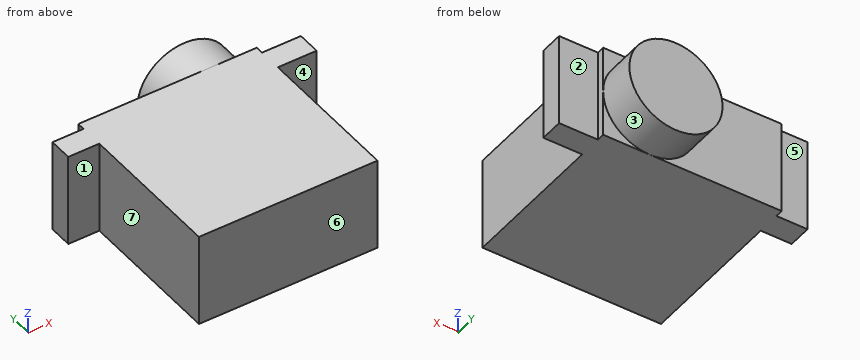
```python
from build123d import *

# Parameters (mm, degrees)
CORPS_SERVO_W      = 23
CORPS_SERVO_H      = 12
BOSS_EXTRU_2_DEPTH = 19
PLAQUE_TROUS_W     = 32
PLAQUE_TROUS_H     = 12
BOSS_EXTRU_3_DEPTH = 3
ESQUISSE5_W        = 23
ESQUISSE5_H        = 12
BOSS_EXTRU_4_DEPTH = 1
ESQUISSE6_R        = 6
BOSS_EXTRU_5_DEPTH = 5


with BuildPart() as part:
    # corps servo → Boss.-Extru.2 (new body)
    with BuildSketch(Plane(origin=(0, 0, 0), x_dir=(1, 0, 0), z_dir=(0, 1, 0))):
        with Locations((11.5, 6)):
            Rectangle(CORPS_SERVO_W, CORPS_SERVO_H)
    extrude(amount=BOSS_EXTRU_2_DEPTH)

    # plaque trous → Boss.-Extru.3 (add)
    with BuildSketch(Plane(origin=(0, 19, 0), x_dir=(1, 0, 0), z_dir=(0, 1, 0))):
        with Locations((12, 6)):
            Rectangle(PLAQUE_TROUS_W, PLAQUE_TROUS_H)
    extrude(amount=BOSS_EXTRU_3_DEPTH)

    # Esquisse5 → Boss.-Extru.4 (add)
    with BuildSketch(Plane(origin=(0, 22, 0), x_dir=(1, 0, 0), z_dir=(0, 1, 0))):
        with Locations((11.5, 6)):
            Rectangle(ESQUISSE5_W, ESQUISSE5_H)
    extrude(amount=BOSS_EXTRU_4_DEPTH)

    # Esquisse6 → Boss.-Extru.5 (add)
    with BuildSketch(Plane(origin=(0, 23, 0), x_dir=(1, 0, 0), z_dir=(0, 1, 0))):
        with Locations((17, 6)):
            Circle(ESQUISSE6_R)
    extrude(amount=BOSS_EXTRU_5_DEPTH)


solid = part.part
```
Geometry: final body of the model. Coordinates: model frame, mm. Face numbers are marked on the shaded views. A direction names the side the tool comes from. Give positions to 0.01 mm unless a question says otherwise; leave off trailing zeros. Write each loop counter-clockwise with the first axis right and the second up, starting at its lowest first coordinate (ties: lowest second). Pieces come first, ordered by that corner, then holes.
1. Reachability of the marked faces 1, 2, 3 and 4 from +Z, -Z, +X, -X, +Y, -Y: full face, straight path, thin tool, end or side. Return the list, or none.
2. Line query: probe 1 along Y at (x, z) = (2.5, -6.25); probe 2 along Y at (x, z) = (24, -0.75). Output: solid intervals per line, ascending.
3. Draft query along Y for the marked faces 5, 6 and 7. Return one class per face: released by +Y, released by -Y, zero draft, split by the parting line, or undercut.
4. Section query A-A, the plane z = -8.25. Return loops of the section in (x, y), then the cut area to 3 significant figures.
5. Section query D-D, the plane z = -10.25. Return loops of the section in (x, y).
6. Section query C-C, the plane x = 19.5. Return loops of the section in (y, z), then the cut area to 3 significant figures.
7. Section query B-B, the plane y = 15.75. Return loops of the section in (x, z).
8. Pin query (flat end, axial travel): P1, Ø3.5, axis at y = 5.5, z = -4, coming from the -X side; P2, Ø4, axis at x = 26.5, z = -4, coming from the +Y side; P3, Ø1, axis at y = 5.5, z = -6, coming from the +X side; P4, Ø1, axis at x = 0.5, y = 17.5, coming from the +Z side. Return the tip coordinate at first contact, or that it passes through.
Computed:
1. face 1: +Z, -Z, -X, -Y
1. face 2: +Z, -Z, +X, +Y
1. face 3: +Y
1. face 4: +Z, -Z, +X, -Y
2. probe 1: y = 0 to 23
2. probe 2: y = 19 to 22
3. face 5: released by +Y
3. face 6: released by -Y
3. face 7: zero draft
4. outline: (-4, 19) - (0, 19) - (0, 0) - (23, 0) - (23, 19) - (28, 19) - (28, 22) - (23, 22) - (23, 23) - (22.56, 23) - (22.56, 28) - (11.44, 28) - (11.44, 23) - (0, 23) - (0, 22) - (-4, 22) - close
4. area: 612 mm2
5. outline: (-4, 19) - (0, 19) - (0, 0) - (23, 0) - (23, 19) - (28, 19) - (28, 22) - (23, 22) - (23, 23) - (21.24, 23) - (21.24, 28) - (12.76, 28) - (12.76, 23) - (0, 23) - (0, 22) - (-4, 22) - close
6. outline: (0, -12) - (23, -12) - (23, -11.45) - (28, -11.45) - (28, -0.55) - (23, -0.55) - (23, 0) - (0, 0) - close
6. area: 331 mm2
7. outline: (0, -12) - (23, -12) - (23, 0) - (0, 0) - close
8. P1: stops at x = 0
8. P2: stops at y = 22
8. P3: stops at x = 23
8. P4: stops at z = 0
